Can you work these out from the model? Positions are in its coordinate system, mm. Face numbers are marked on the shaded views. A direction names the side the tool comes from. Round coordinates to 2 decimals unless told otherwise and drop trailing zeros. Write each loop counter-clockwise with the first axis right and the second up, starting at its lowest first coordinate (ties: lowest second). Pieces come first, ordered by that corner, then holes. Notation, with made-up numbers: (-37, 31) - (-5, 31) arc R27 cw to (-5, 48) - close; hole circle Ø1 at (-4.5, 46). An arc over 180 degrees is marked (long way). One line per item, written item: value. Start each with the question number.
(1) On a 3-axis mill with a long thin cutter (end or side, diameter ignored), from which of +Z, -Z, +X, -X, +Y, -Y can I reach the whole of each face in a straight line? I mean the marked faces 1 and 2. Say none if no direction works.
(2) I want a section at A-A on z = -4.5. List the corners of the cut face in (x, y) for me.
(3) If I drill on L1, parallel to X at y = 6, z = -3.2; L2, parallel to Y at x = -12.5, z = -4.3; L3, parallel to X at y = 6.5, z = -3.75, over which ranges is the centre line in solid material (lowest first)? Write a range as from..to.
(4) I want a section at C-C on y = 4. List the corners of the cut face in (x, z) for me, plus the area to 3 significant figures.
(5) I want a section at B-B on x = -12.5. List the corners of the cut face in (y, z) for me.
(6) I'm going to push flat-ended pins straight in: pin 1 Ø2 at (y, z) = (-2, 0) entering from +X; pin 2 Ø1 at (x, y) = (4.5, -16) entering from -Z; pin 3 Ø2.5 at (x, y) = (-13, -6.5) entering from -Z; pin 4 Ø0.5 at (y, z) = (-21, 3.5) entering from +X. Where does each tip first touch, or does it pass through?
(7) Thinking about a two-plate mould opening in X: for the marked faces 3, 4 and 5, which applies, +X half, -X half, draft (parallel to the pull), parting line (faces both ways), or undercut?
Autodesk Inventor part; units mm, degrees
ref_plane "YZ Plane" through (0, 0, 0) normal (1, 0, 0) x (0, 1, 0)
ref_plane "XZ Plane" through (0, 0, 0) normal (0, 1, 0) x (-1, 0, 0)
ref_plane "XY Plane" through (0, 0, 0) normal (0, 0, 1) x (1, 0, 0)
sketch "Náčrt1" plane through (0, 0, 0) normal (0, 0, 1) x (1, 0, 0)
  arc A0 (10.1858, -15.4434) -> (-9.4468, -15.9062) centre (0, 0) ccw
  line L0 (7.4894, -20.4521) -> (7.4894, -21.5)
  line L1 (7.4894, -21.5) -> (-6.5106, -21.5)
  line L2 (-6.5106, -21.5) -> (-6.5106, -21.065)
  line L3 (0, -18.5) -> (7.4894, -21.5) construction
  line L4 (0, -18.5) -> (-6.5106, -21.5) construction
  line L5 (0, 18.5) -> (0, -37.4433)
  arc A1 (-6.5106, -21.065) -> (-9.4468, -15.9062) centre (-12.5106, -21.065) ccw
  arc A2 (10.1858, -15.4434) -> (7.4894, -20.4521) centre (13.4894, -20.4521) ccw
  line L6 (-12.5, 6) -> (12.5, 6)
  line L7 (12.5, 6) -> (12.5, -6)
  line L8 (12.5, -6) -> (-12.5, -6)
  line L9 (-12.5, -6) -> (-12.5, 6)
  line L10 (-12.5, 6) -> (12.5, -6) construction
  line L11 (12.5, 6) -> (-12.5, -6) construction
  circle A3 centre (-12.5, 6) radius 1.5
  circle A4 centre (12.5, 6) radius 1.5
  circle A5 centre (12.5, -6) radius 1.5
  circle A6 centre (-12.5, -6) radius 1.5
  circle A7 centre (-12.5, 6) radius 2.75
  circle A8 centre (12.5, 6) radius 2.75
  circle A9 centre (12.5, -6) radius 2.75
  circle A10 centre (-12.5, -6) radius 2.75
  point P0 (7.4894, -16.9162)
  point P1 (-6.5106, -17.3165)
  dimension "d0" = 37
  dimension "d1" = 14
  dimension "d2" = 21.5
  dimension "d3" = 6
  dimension "d4" = 25
  dimension "d5" = 12
  dimension "d6" = 3
  dimension "d7" = 3
  dimension "d8" = 3
  dimension "d9" = 3
  dimension "d10" = 5.5
  dimension "d11" = 5.5
  dimension "d12" = 5.5
  dimension "d13" = 5.5
extrude "Vysunutí1" add sketch "Náčrt1" along normal blind 5
extrude "Vysunutí2" add sketch "Náčrt1" against normal blind 6 contours A7 L9 A3 L6 | L6 A3 L9 A7 | A8 L7 A4 L6 | L6 A4 L7 A8 | A9 L7 A5 L8 | L8 A5 L7 A9 | A10 L9 A6 L8 | L8 A6 L9 A10
thread "Závit1"
thread "Závit2"
thread "Závit3"
thread "Závit4"
properties part number "Disp"
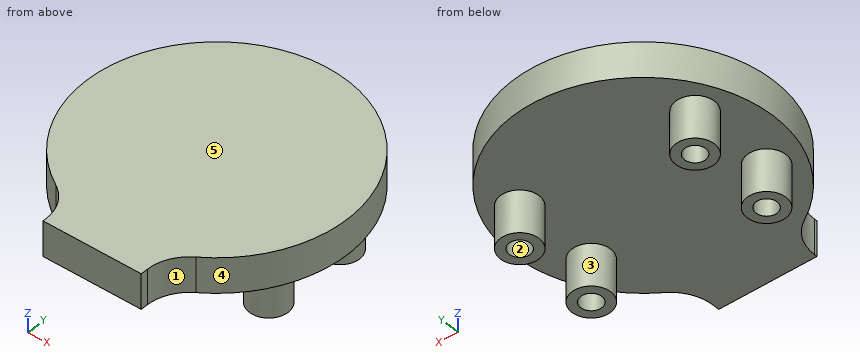
Established:
1. face 1: +Z, -Z, +X, -Y
1. face 2: -Z
2. outline: circle Ø5.5 at (-12.5, -6); circle Ø5.5 at (-12.5, 6); circle Ø5.5 at (12.5, -6); circle Ø5.5 at (12.5, 6); hole circle Ø3 at (-12.5, -6); hole circle Ø3 at (-12.5, 6); hole circle Ø3 at (12.5, -6); hole circle Ø3 at (12.5, 6)
3. L1: -15.25..-14, -11..-9.75, 9.75..11, 14..15.25
3. L2: -8.75..-7.5, -4.5..-3.25, 3.25..4.5, 7.5..8.75
3. L3: -15.2..-13.91, -11.09..-9.8, 9.8..11.09, 13.91..15.2
4. outline: (-18.06, 0) - (-14.39, 0) - (-14.39, -6) - (-10.61, -6) - (-10.61, 0) - (10.61, 0) - (10.61, -6) - (14.39, -6) - (14.39, 0) - (18.06, 0) - (18.06, 5) - (-18.06, 5) - close
4. area: 226 mm2
5. outline: (-13.64, 0) - (-8.75, 0) - (-8.75, -6) - (-7.5, -6) - (-7.5, 0) - (-4.5, 0) - (-4.5, -6) - (-3.25, -6) - (-3.25, 0) - (3.25, 0) - (3.25, -6) - (4.5, -6) - (4.5, 0) - (7.5, 0) - (7.5, -6) - (8.75, -6) - (8.75, 0) - (13.64, 0) - (13.64, 5) - (-13.64, 5) - close
6. pin 1: x = 18.47
6. pin 2: z = 0
6. pin 3: z = -6
6. pin 4: x = 7.49
7. face 3: undercut
7. face 4: parting line
7. face 5: draft
